```python
from build123d import *

# Parameters (mm, degrees)
SKETCH1_W           = 431.8
SKETCH1_H           = 88.9
BOSS_EXTRUDE1_DEPTH = 22.225
SKETCH2_W           = 15.875
SKETCH2_H           = 69.85
BOSS_EXTRUDE2_DEPTH = 50.8
SKETCH3_R           = 4.7625
CUT_EXTRUDE1_DEPTH  = 273.056003253
SKETCH5_R           = 6.35
CUT_EXTRUDE3_DEPTH  = 283.003635836


with BuildPart() as part:
    # Sketch1 → Boss-Extrude1 (new, symmetric)
    with BuildSketch(Plane.XY):
        Rectangle(SKETCH1_W, SKETCH1_H)
    extrude(amount=BOSS_EXTRUDE1_DEPTH, both=True)

    # Sketch2 → Boss-Extrude2 (add)
    with BuildSketch(Plane(origin=(215.9, 0, 0), x_dir=(0, 0, -1), z_dir=(1, 0, 0))):
        with Locations((0, -9.525)):
            Rectangle(SKETCH2_W, SKETCH2_H)
    boss_extrude2 = extrude(amount=BOSS_EXTRUDE2_DEPTH)

    # Sketch3 → Cut-Extrude1 (cut, through all)
    with BuildSketch(Plane.XY.offset(7.9375)):
        with Locations((241.3, 14.2875)):
            Circle(SKETCH3_R)
        with Locations((241.3, -33.3375)):
            Circle(SKETCH3_R)
    cut_extrude1 = extrude(amount=-CUT_EXTRUDE1_DEPTH, mode=Mode.SUBTRACT)

    # Mirror1: Boss-Extrude2, Cut-Extrude1 across plane
    add(boss_extrude2.mirror(Plane(origin=(0, 0, 0), x_dir=(0, 0, 1), z_dir=(1, 0, 0))))
    add(cut_extrude1.mirror(Plane(origin=(0, 0, 0), x_dir=(0, 0, 1), z_dir=(1, 0, 0))), mode=Mode.SUBTRACT)

    # Sketch5 → Cut-Extrude3 (cut, through all)
    with BuildSketch(Plane(origin=(0, 44.45, 0), x_dir=(1, 0, 0), z_dir=(0, 1, 0))):
        with Locations(Location((-152.4, 0, 0), (0, 0, 180))):
            Circle(SKETCH5_R)
        with Locations(Location((152.4, 0, 0), (0, 0, 180))):
            Circle(SKETCH5_R)
    extrude(amount=-CUT_EXTRUDE3_DEPTH, mode=Mode.SUBTRACT)


solid = part.part
```
Source: CAD feature listing. Evaluate the final solid. Frame: model axes, mm. A direction names the side the tool comes from. Coordinates: 2 decimals unless noted, no trailing zeros. Loops run counter-clockwise (first coordinate to the right, second up) from the corner with the lowest first, then second, coordinate; pieces in that order, holes last. Notation, with made-up numbers: M -8,69.25 L 20,69.25 A35 cw 20,107.25 Z; hole C 5,43 d10. An arc over 180 degrees is marked long. Put each result on its own line as item: value. Start each with the question number.
1) Cut plane A-A on x = 152.4. Return the cut outline in (y, z) (3 decimals), then the cut area to 3 significant figures.
2) Pull-direction query (Y, two-part tool) for faces 4 (the face through (215.9, -1, 10)), 5 (the face through (245.84, 15.72, 0.11)), 6 (the face through (-3, 44.45, 0)), 7 (the face through (-245.7, -35.16, 0.11)); classes: pulls with the +Y half, pulls with the -Y half, needs draft (parallel to the pull), parting line crosses it, or undercut.
3) Contact query for flat-ended pins moving along their axis: pin 1 Ø1 at (y, z) = (-18.5, -12) entering from -X; pin 2 Ø11 at (x, y) = (241.3, -33.34) entering from -Z; pin 3 Ø2 at (y, z) = (-25.5, -10) entering from +X. Output: stop coordinate, or through.
4) Reachability of faces 1 (the face through (241, -10, -7.938)), 2 (the face through (241, 25.4, 0)), 3 (the face through (-241, 25.4, 0)) from +Z, -Z, +X, -X, +Y, -Y: full face, straight path, thin tool, end or side. Return the list, or none.
5) Ray query, L1, parallel to Y at x = 241.3, z = 1.5 (3 decimals); L2, parallel to X at y = -41, z = -4; L3, parallel to X at y = 11.5, z = 3.5. Return the intervals inside material, ascending. Write a range as from..to.
6) Cut plane B-B on x = 241.3. Give the number of separate pieces and of enclosed holes in the cut face, then the cut area to 3 significant figures.
The answers:
1. outline: M -44.45,-22.225 L 44.45,-22.225 L 44.45,-6.35 L -44.45,-6.35 Z; M -44.45,6.35 L 44.45,6.35 L 44.45,22.225 L -44.45,22.225 Z
1. area: 2,820 mm²
2. face 4: needs draft
2. face 5: undercut
2. face 6: pulls with the +Y half
2. face 7: undercut
3. pin 1: stops at x = -215.9
3. pin 2: stops at z = -7.94
3. pin 3: stops at x = 215.9
4. face 1: -Z, +X, +Y, -Y
4. face 2: +Z, -Z, +X, +Y
4. face 3: +Z, -Z, -X, +Y
5. L1: y = -44.45..-38.1, -28.575..9.525, 19.05..25.4
5. L2: x = -266.7..-157.33, -147.47..147.47, 157.33..266.7
5. L3: x = -266.7..-245.16, -237.44..-157.7, -147.1..147.1, 157.7..237.44, 245.16..266.7
6. separate pieces: 3
6. enclosed holes: 0
6. area: 806 mm²
